```python
from build123d import *

# Parameters (mm, degrees)
F1_DEPTH = 30
F2_W     = 23
F2_H     = 24
F3_DEPTH = 20.001


with BuildPart() as f1:
    # F0 (on Front) → F1 (new body)
    with BuildSketch(Plane.XZ):
        with BuildLine():
            Line((0, 20), (0, 0))
            Line((0, 0), (48, 0))
            ThreePointArc((48, 0), (55.071068, 2.928932), (58, 10))
            Line((58, 10), (58, 25))
            Line((58, 25), (48, 25))
            Line((48, 25), (48, 20))
            Line((48, 20), (39, 20))
            Line((39, 20), (39, 23))
            Line((39, 23), (36, 23))
            Line((36, 23), (36, 20))
            Line((36, 20), (9, 20))
            Line((9, 20), (9, 23))
            Line((9, 23), (6, 23))
            Line((6, 23), (6, 20))
            Line((6, 20), (0, 20))
        make_face()
    extrude(amount=F1_DEPTH)

    # F2 (on face) → F3 (cut, through all)
    with BuildSketch(Plane.XY.offset(20)):
        with Locations((22.5, -15)):
            Rectangle(F2_W, F2_H)
    extrude(amount=-F3_DEPTH, mode=Mode.SUBTRACT)


solid = f1.part
```
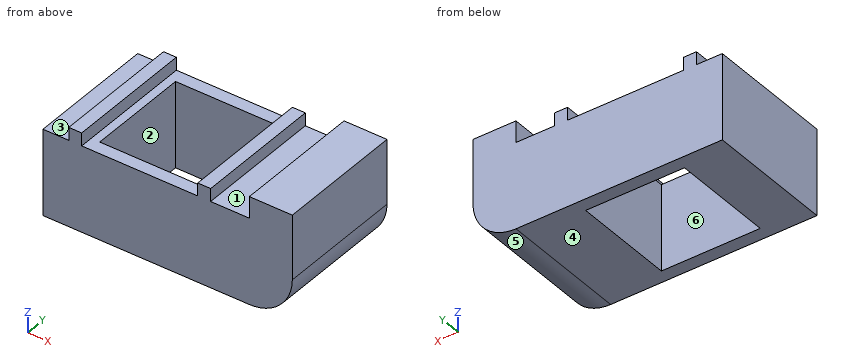
For this review, take the finished solid that the model builds, in its own axes (mm). Face numbers are marked on the shaded views. A direction names the side the tool comes from. Coordinates: 2 decimals unless noted, no trailing zeros. Loops run counter-clockwise (first coordinate to the right, second up) from the corner with the lowest first, then second, coordinate; pieces in that order, holes last. Notation, with made-up numbers: (7, -3.75) -> (51, -3.75) arc R14 cw to (51, 1.25) -> close; hole circle Ø11 at (34, 25.5). An arc over 180 degrees is marked (long way). Return JSON: item names as keys, results as strings. Group by question number.
(1) Consider section C-C, the plane y = -9. Give the boundary of the cut face in (x, z), plus the area to 3 significant figures.
(2) Consider section A-A, the plane x = 21.5. Give the boundary of the cut face in (y, z), plus the area to 3 significant figures.
(3) To check wall thickness, follow L1, parallel to Y at x = 24, z = 2; L2, parallel to X at y = -17.5, z = 14.5; L3, parallel to X at y = -12.25, z = 9. State the ranges of each line that lie inside material, in increasing order.
(4) Tool access review of the marked faces 1, 2 and 3: name each direction out of +Z, -Z, +X, -X, +Y, -Y from which nothing blocks a thin tool from reaching the whole face with its end or side.
(5) Consider section B-B, the plane z = 11.5. Give the boundary of the cut face in (x, y).
(6) For pin 1 Ø6 at (x, z) = (19, 6.5) entering from +Y; pin 2 Ø13.5 at (x, y) = (28.5, -12.5) entering from +Z; pin 3 Ø2.5 at (y, z) = (-11, 22.5) entering from -X; pin 4 Ø2.5 at (x, y) = (7.5, -13) entering from +Z, all flat-tipped, find the tip position at first contact; note any pin that passes through.
(7) Consider section D-D, the plane z = 21. Give the boundary of the cut face in (x, y).
(8) Mouldability with a two-part tool opening along X and no side actions: class the marked faces 4, 5 and 6 as pulls with the +X half, pulls with the -X half, needs draft (parallel to the pull), parting line crosses it, or undercut.
Results below:
{
 "1": {"outline": "(0, 0) -> (11, 0) -> (11, 20) -> (9, 20) -> (9, 23) -> (6, 23) -> (6, 20) -> (0, 20) -> close; (34, 0) -> (48, 0) arc R10 ccw to (58, 10) -> (58, 25) -> (48, 25) -> (48, 20) -> (39, 20) -> (39, 23) -> (36, 23) -> (36, 20) -> (34, 20) -> close", "area": "747 mm2"},
 "2": {"outline": "(-30, 0) -> (-27, 0) -> (-27, 20) -> (-30, 20) -> close; (-3, 0) -> (0, 0) -> (0, 20) -> (-3, 20) -> close", "area": "120 mm2"},
 "3": {"L1": "y = -30 to -27, -3 to 0", "L2": "x = 0 to 11, 34 to 58", "L3": "x = 0 to 11, 34 to 57.95"},
 "4": {"face 1": "+Z, +Y, -Y", "face 2": "+Z, -Z", "face 3": "+Z, -X, +Y, -Y"},
 "5": {"outline": "(0, -30) -> (58, -30) -> (58, 0) -> (0, 0) -> close; hole (11, -27) -> (34, -27) -> (34, -3) -> (11, -3) -> close"},
 "6": {"pin 1": "stops at y = 0", "pin 2": "stops at z = 20", "pin 3": "stops at x = 6", "pin 4": "stops at z = 23"},
 "7": {"outline": "(6, -30) -> (9, -30) -> (9, 0) -> (6, 0) -> close; (36, -30) -> (39, -30) -> (39, 0) -> (36, 0) -> close; (48, -30) -> (58, -30) -> (58, 0) -> (48, 0) -> close"},
 "8": {"face 4": "needs draft", "face 5": "pulls with the +X half", "face 6": "undercut"}
}
